The drawing under review shows one solid part. Ordinate dimensions are in mm from its lowest x, y, z. Coordinates: 2 decimals unless noted, no trailing zeros. Write each loop counter-clockwise with the first axis right and the second up, starting at its lowest first coordinate (ties: lowest second). Pieces come first, ordered by that corner, then holes.
1) We need section B-B on z = 1.5. Write out the cut boundary in (x, y).
2) We need section C-C on x = 8.5. Write out the cut boundary in (y, z).
3) We need section A-A on y = 60. Write out the cut boundary in (x, z), then the cut area to 3 significant figures.
4) To check wall thickness, follow line 1 along Z through (x, y) = (5.75, 136); line 2 along X through (y, z) = (27, 5.5); line 3 along Z through (x, y) = (2, 125.5). State the ranges of each line that lie inside material, in increasing order.
5) Insertion check: P1, Ø3, axis at x = 8, z = 2, coming from the -Y side. The pin has a flat end and moves straight along its axis. Give the tip position at first contact, or say it passes through.
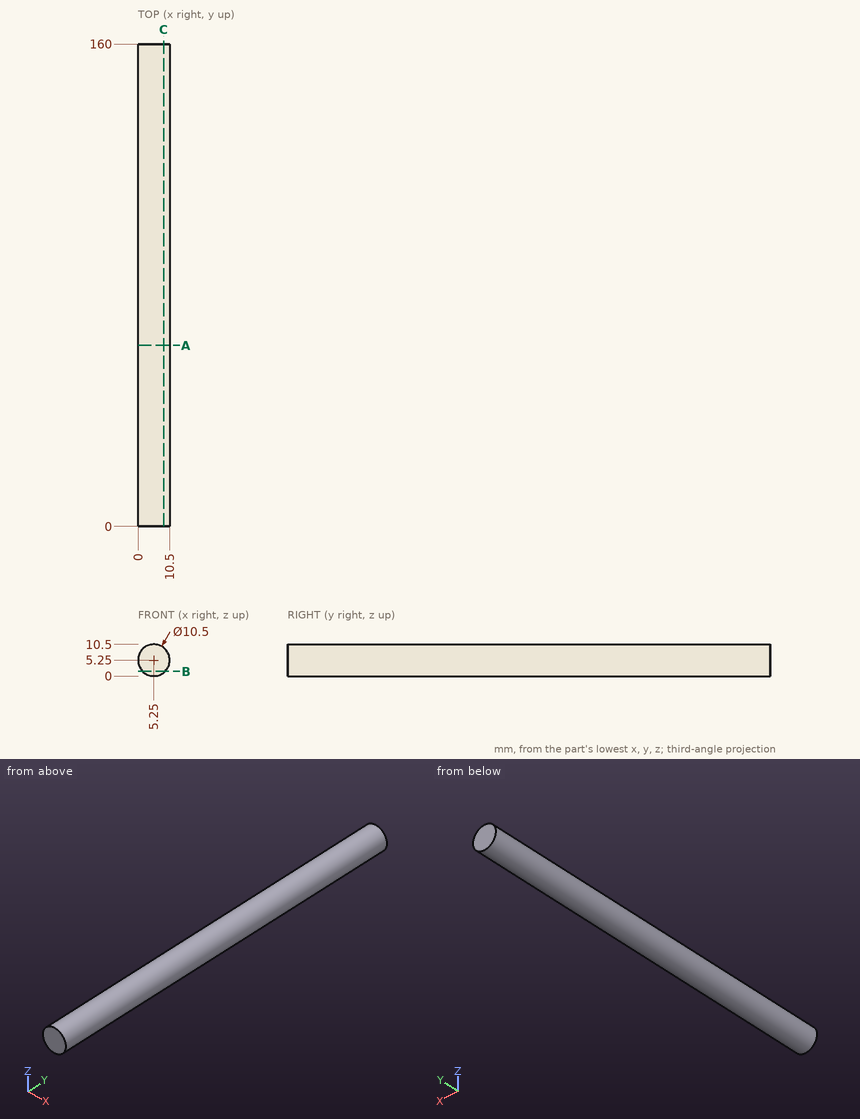
Result:
1. outline: (1.58, 0) - (8.92, 0) - (8.92, 160) - (1.58, 160) - close
2. outline: (0, 1.13) - (160, 1.13) - (160, 9.37) - (0, 9.37) - close
3. outline: circle Ø10.5 at (5.25, 5.25)
3. area: 86.6 mm2
4. line 1: z = 0.02 to 10.48
4. line 2: x = 0.01 to 10.49
4. line 3: z = 1.13 to 9.37
5. P1: stops at y = 0
